Autodesk Inventor part; units mm, degrees
ref_plane "YZ Plane" through (0, 0, 0) normal (1, 0, 0) x (0, 1, 0)
ref_plane "XZ Plane" through (0, 0, 0) normal (0, 1, 0) x (-1, 0, 0)
ref_plane "XY Plane" through (0, 0, 0) normal (0, 0, 1) x (1, 0, 0)
sketch "Sketch1" plane through (0, 0, 0) normal (0, 0, 1) x (1, 0, 0)
  line L0 (-6.3269, 6.7325) -> (69.8731, 6.7325)
  line L1 (69.8731, 6.7325) -> (69.8731, -69.4675)
  line L2 (69.8731, -69.4675) -> (-6.3269, -69.4675)
  line L3 (-6.3269, -69.4675) -> (-6.3269, 6.7325)
  line L4 (-6.3269, 6.7325) -> (69.8731, -69.4675) construction
  line L5 (69.8731, 6.7325) -> (-6.3269, -69.4675) construction
  circle A0 centre (31.7731, -31.3675) radius 4.7625
  circle A1 centre (63.9041, 0.7635) radius 1.8161
  circle A2 centre (63.9041, -63.4985) radius 1.8161
  circle A3 centre (-0.3579, -63.4985) radius 1.8161
  circle A4 centre (-0.3579, 0.7635) radius 1.8161
  line L6 (12.7231, -50.4175) -> (50.8231, -50.4175) construction
  line L7 (50.8231, -50.4175) -> (50.8231, -12.3175) construction
  line L8 (50.8231, -12.3175) -> (12.7231, -12.3175) construction
  line L9 (12.7231, -12.3175) -> (12.7231, -50.4175) construction
  line L10 (12.7231, -50.4175) -> (50.8231, -12.3175) construction
  line L11 (50.8231, -50.4175) -> (12.7231, -12.3175) construction
  circle A5 centre (19.416, -19.0104) radius 2.0193
  circle A6 centre (44.1302, -19.0104) radius 2.0193
  circle A7 centre (19.416, -43.7246) radius 2.0193
  circle A8 centre (44.1302, -43.7246) radius 2.0193
  dimension "d0" = 76.2
  dimension "d1" = 76.2
  dimension "d2" = 9.525
  dimension "d4" = 3.6322
  dimension "d5" = 3.6322
  dimension "d6" = 3.6322
  dimension "d7" = 3.6322
  dimension "d11" = 38.1
  dimension "d12" = 38.1
  dimension "d13" = 4.0386
  dimension "d14" = 4.0386
  dimension "d15" = 4.0386
  dimension "d16" = 4.0386
  dimension "d17" = 24.7142
  dimension "d18" = 64.262
extrude "Extrusion1" add sketch "Sketch1" along normal blind 11.43
sketch "Sketch2" plane through (0, 0, 11.43) normal (0, 0, 1) x (1, 0, 0)
  circle A0 centre (31.7731, -31.3675) radius 4.7625 construction
  line L0 (27.0106, -31.3675) -> (38.4406, -31.3675) construction
  line L1 (38.4406, -31.3675) -> (38.4406, -29.5895) construction
  line L2 (38.4406, -29.5895) -> (34.9614, -29.5895)
  line L3 (34.9614, -29.5895) -> (34.9614, -33.8756)
  line L4 (34.9614, -33.8756) -> (38.4406, -33.8756)
  line L5 (38.4406, -33.8756) -> (38.4406, -29.5895)
  point P0 (0, 0)
  dimension "d21" = 11.43
  dimension "d22" = 1.778
extrude "Extrusion2" cut sketch "Sketch2" along normal through all both and the other way through all
sketch "Sketch3" plane through (0, 0, 11.43) normal (0, 0, 1) x (1, 0, 0)
  line L0 (38.4406, -33.8756) -> (35.8216, -33.8756)
  line L1 (38.4406, -29.5895) -> (35.8216, -29.5895)
  line L2 (35.8216, -33.8756) -> (38.4406, -33.8756)
  line L3 (38.4406, -33.8756) -> (38.4406, -29.5895)
  arc A0 (35.8216, -33.8756) -> (36.1912, -29.5895) centre (31.7731, -31.3675) ccw
  line L4 (35.8216, -33.8756) -> (38.4406, -33.8756)
  line L5 (38.4406, -29.5895) -> (36.1912, -29.5895)
  line L6 (38.4406, -29.5895) -> (36.1912, -29.5895)
  point P0 (0, 0)
  point P1 (31.7731, -31.3675)
extrude "Extrusion3" add sketch "Sketch3" against normal up to surface (11.43 mm away)
sketch "Sketch4" plane through (0, 0, 11.43) normal (0, 0, 1) x (1, 0, 0)
  circle A0 centre (31.7731, -31.3675) radius 4.7625 construction
  line L0 (27.0106, -31.3675) -> (38.4406, -31.3675) construction
  line L1 (38.4406, -31.3675) -> (38.4406, -29.4625) construction
  line L2 (38.4406, -29.4625) -> (38.4406, -33.2725)
  line L3 (38.4406, -33.2725) -> (36.138, -33.2725)
  line L4 (38.4406, -29.4625) -> (36.138, -29.4625)
  arc A1 (36.138, -33.2725) -> (36.138, -29.4625) centre (31.7731, -31.3675) ccw
  point P0 (0, 0)
  dimension "d27" = 11.43
  dimension "d28" = 1.905
  dimension "d29" = 3.81
extrude "Extrusion4" cut sketch "Sketch4" against normal up to surface (11.43 mm away)
sketch "Sketch5" plane through (0, 0, 11.43) normal (0, 0, 1) x (1, 0, 0)
  line L0 (38.4406, -33.2725) -> (38.4406, -29.4625) construction
  line L1 (38.4406, -29.4625) -> (38.4406, -27.0625) construction
  line L2 (38.4406, -33.2725) -> (38.4406, -35.6725) construction
  line L3 (38.4406, -35.6725) -> (37.2928, -35.6725)
  line L4 (37.2928, -35.6725) -> (37.2928, -36.8725)
  line L5 (37.2928, -36.8725) -> (38.4406, -36.8725)
  line L6 (38.4406, -36.8725) -> (38.4406, -35.6725)
  line L7 (38.4406, -27.0625) -> (37.2928, -27.0625)
  line L8 (37.2928, -27.0625) -> (37.2928, -25.8625)
  line L9 (37.2928, -25.8625) -> (38.4406, -25.8625)
  line L10 (38.4406, -25.8625) -> (38.4406, -27.0625)
  arc A0 (36.138, -29.4625) -> (36.138, -33.2725) centre (31.7731, -31.3675) ccw
  line L11 (36.138, -29.4625) -> (38.4406, -29.4625) construction
  line L12 (38.4406, -29.4625) -> (40.8406, -29.4625) construction
  line L13 (40.8406, -29.4625) -> (42.0406, -29.4625)
  line L14 (42.0406, -29.4625) -> (42.0406, -33.2725)
  line L15 (42.0406, -33.2725) -> (40.8406, -33.2725)
  line L16 (40.8406, -33.2725) -> (40.8406, -29.4625)
  point P0 (0, 0)
  dimension "d32" = 2.4
  dimension "d33" = 2.4
  dimension "d34" = 1.2
  dimension "d35" = 1.2
  dimension "d36" = 7
  dimension "d37" = 2.4
  dimension "d38" = 1.2
extrude "Extrusion5" cut sketch "Sketch5" against normal blind 25.4
sketch "Sketch6" plane through (0, 0, 11.43) normal (0, 0, 1) x (1, 0, 0)
  point P0 (0, 0)
sketch "Sketch7" plane through (0, 0, 11.43) normal (0, 0, 1) x (1, 0, 0)
  arc A0 (36.138, -29.4625) -> (36.138, -33.2725) centre (31.7731, -31.3675) ccw
  circle A1 centre (31.7731, -31.3675) radius 5.3
  point P0 (0, 0)
  dimension "d41" = 10.6
extrude "Extrusion6" cut sketch "Sketch7" against normal through all
properties part number "armmount"
Model file for the job. Use its own axes, mm. A direction names the side the tool comes from. Give positions to 0.01 mm unless a question says otherwise; leave off trailing zeros. Order: outer loops, then holes, each group sorted by start corner. A loop starts at its lowest first (then second) coordinate and runs counter-clockwise, first axis right, second up.
1) Saw through at A-A, the plane x = 29.5. Write the cut outline in (y, z), then the cut area to 3 significant figures.
2) 3-axis set-ups, long thin cutter, end or side, ignore diameter. For faces 1 (the flat face through (31, -22, 11.43)), 2 (the flat face through (38, -33.272, 6)): which of +Z, -Z, +X, -X, +Y, -Y reach the whole face in a straight line?
3) Pin check, flat tip, straight feed: pin 1 (2.5 mm diameter, centred on x = 19.42, y = -19.01, fed in from +Z). Stop position of the tip, or through.
4) Wall check: probe 1 along X at (y, z) = (-19, 10.5); probe 2 along Y at (x, z) = (44, 9.25); probe 3 along Y at (x, z) = (43.5, 1.75). Give the ranges that are in metal, low to high.
5) Mould opens along Y. For faces 3 (the cylindrical face through (26.477, -31.162, 5.795)), 4 (the flat face through (31, 6.732, 6)), 5 (the flat face through (40.841, -31, 6)), 6 (the flat face through (31, -22, 0)) say: +Y half, -Y half, draft (parallel to the pull), parting line (faces both ways), or undercut.
6) Saw through at C-C, the plane y = -18. Write the cut outline in (x, z), then the cut area to 3 significant figures.
7) Saw through at B-B, the plane z = 8. Count the separate pieces of the cut face and the enclosed holes in it, then the cut area to 3 significant figures.
Computed:
1. outline: (-69.47, 0) - (-36.16, 0) - (-36.16, 11.43) - (-69.47, 11.43) - close; (-26.58, 0) - (6.73, 0) - (6.73, 11.43) - (-26.58, 11.43) - close
1. area: 762 mm2
2. face 1: +Z, +X, -X, +Y, -Y
2. face 2: +Z, -Z
3. pin 1: passes through
4. probe 1: x = -6.33 to 17.4, 21.44 to 42.11, 46.15 to 69.87
4. probe 2: y = -69.47 to -45.74, -41.71 to -21.03, -17 to 6.73
4. probe 3: y = -69.47 to -45.64, -41.81 to -20.93, -17.09 to 6.73
5. face 3: undercut
5. face 4: +Y half
5. face 5: undercut
5. face 6: draft
6. outline: (-6.33, 0) - (17.67, 0) - (17.67, 11.43) - (-6.33, 11.43) - close; (21.16, 0) - (42.38, 0) - (42.38, 11.43) - (21.16, 11.43) - close; (45.88, 0) - (69.87, 0) - (69.87, 11.43) - (45.88, 11.43) - close
6. area: 791 mm2
7. separate pieces: 1
7. enclosed holes: 12
7. area: 5,610 mm2
